Geometry check sheet. Reference: the model listing, model coordinates, mm. A direction names the side the tool comes from. Round coordinates to 2 decimals unless told otherwise and drop trailing zeros. Loops run counter-clockwise (first coordinate to the right, second up) from the corner with the lowest first, then second, coordinate; pieces in that order, holes last. Notation, with made-up numbers: (-11, 30) - (18, 30) arc R10 cw to (18, 49) - close; hole circle Ø10 at (44, -31.75). An arc over 180 degrees is marked (long way). Write item = value, one per line.
```python
from build123d import *

# Parameters (mm, degrees)
F0_W     = 123.5331967473
F0_H     = 85.607599467
F0_W_2   = 110.4088798165
F0_H_2   = 66.8058078736
F1_DEPTH = 80.518
F2_W     = 42.3468332738
F2_H     = 27.7133138709
F3_DEPTH = 85.608599467
F4_R     = 14.5797051929
F5_DEPTH = 123.5341967473


with BuildPart() as f1:
    # F0 (on Top) → F1 (new body)
    with BuildSketch(Plane.XY):
        with Locations((-0.5623660982, 9.3691665679)):
            Rectangle(F0_W, F0_H)
        with Locations((-0.2685114741, 11.0694328323)):
            Rectangle(F0_W_2, F0_H_2, mode=Mode.SUBTRACT)
    extrude(amount=F1_DEPTH)

    # F2 (on face) → F3 (cut, through all)
    with BuildSketch(Plane.XZ.offset(33.4346331656)):
        with Locations((2.2117001936, 66.6613430645)):
            Rectangle(F2_W, F2_H)
    extrude(amount=-F3_DEPTH, mode=Mode.SUBTRACT)

    # F4 (on face) → F5 (cut, through all)
    with BuildSketch(Plane.YZ.offset(61.2042322755)):
        with Locations((0, 34.6741601825)):
            Circle(F4_R)
    extrude(amount=-F5_DEPTH, mode=Mode.SUBTRACT)


solid = f1.part
```
(1) Gauge pin test, flat end, axial feed: pin 1 (6 mm diameter, centred on x = 5, y = 49, fed in from +Z). Record the tip position at first contact, or that the pin passes through.
Answers follow:
pin_1 = 52.8
(2) Scan lines: L1, parallel to Z at x = -60, y = 0; L2, parallel to Y at x = -36.5, z = 19.5; L3, parallel to X at y = 44, z = 9.5. Record each from-to range of solid material in increasing order. Write a range as [from, to].
Answers follow:
L1 = [0, 20.09], [49.25, 80.52]
L2 = [-33.43, -22.33], [44.47, 52.17]
L3 = [-62.33, -55.47], [54.94, 61.2]
(3) Section check B-B (x = 8). Enter the section's corners in (y, z), then the cut area to 3 significant figures.
Answers follow:
outline = (-33.43, 0) - (-22.33, 0) - (-22.33, 52.8) - (-33.43, 52.8) - close; (44.47, 0) - (52.17, 0) - (52.17, 52.8) - (44.47, 52.8) - close
area = 993 mm²
(4) Section check C-C (z = 74). Enter the section's corners in (x, y), then the cut area to 3 significant figures.
Answers follow:
outline = (-62.33, -33.43) - (-18.96, -33.43) - (-18.96, -22.33) - (-55.47, -22.33) - (-55.47, 44.47) - (-18.96, 44.47) - (-18.96, 52.17) - (-62.33, 52.17) - close; (23.39, -33.43) - (61.2, -33.43) - (61.2, 52.17) - (23.39, 52.17) - (23.39, 44.47) - (54.94, 44.47) - (54.94, -22.33) - (23.39, -22.33) - close
area = 2,400 mm²
(5) Section check D-D (y = -25). Enter the section's corners in (x, z), then the cut area to 3 significant figures.
Answers follow:
outline = (-62.33, 0) - (61.2, 0) - (61.2, 80.52) - (23.39, 80.52) - (23.39, 52.8) - (-18.96, 52.8) - (-18.96, 80.52) - (-62.33, 80.52) - close
area = 8,770 mm²
(6) Section check A-A (y = 0). Enter the section's corners in (x, z), then the cut area to 3 significant figures.
Answers follow:
outline = (-62.33, 0) - (-55.47, 0) - (-55.47, 20.09) - (-62.33, 20.09) - close; (-62.33, 49.25) - (-55.47, 49.25) - (-55.47, 80.52) - (-62.33, 80.52) - close; (54.94, 0) - (61.2, 0) - (61.2, 20.09) - (54.94, 20.09) - close; (54.94, 49.25) - (61.2, 49.25) - (61.2, 80.52) - (54.94, 80.52) - close
area = 674 mm²
(7) Set-up check for faces 4 (the flat face through (-55.473, 18, 40)), 5 (the flat face through (-18.962, -28, 66)), 6 (the flat face through (-62.329, 18, 40)): record each of +Z, -Z, +X, -X, +Y, -Y from which the full face is reachable in a straight line by a thin tool's end or side.
Answers follow:
face_4 = +Z, -Z
face_5 = +Z, +Y, -Y
face_6 = +Z, -Z, -X, +Y, -Y
(8) Mould release check, pull along Z, two halves, no side actions. Record for faces 1 (the flat face through (23.385, 48, 66)), 2 (the flat face through (2, 48, 52.805)), 3 (the cylindrical face through (-58.85, -3.16, 20.44)): pulls with the +Z half, pulls with the -Z half, needs draft (parallel to the pull), parting line crosses it, or undercut.
Answers follow:
face_1 = needs draft
face_2 = pulls with the +Z half
face_3 = undercut
